The listing builds one solid part. Answer for the finished solid, in the listing's coordinates (mm). Coordinates: 2 decimals unless noted, no trailing zeros. Loops run counter-clockwise (first coordinate to the right, second up) from the corner with the lowest first, then second, coordinate; pieces in that order, holes last. Notation, with made-up numbers: (-37, -4.5) - (16, -4.5) arc R35 ccw to (16, 33.5) - close; hole circle Ø11 at (66, 9.5). An arc over 180 degrees is marked (long way). One line per question, with ' | ' between items.
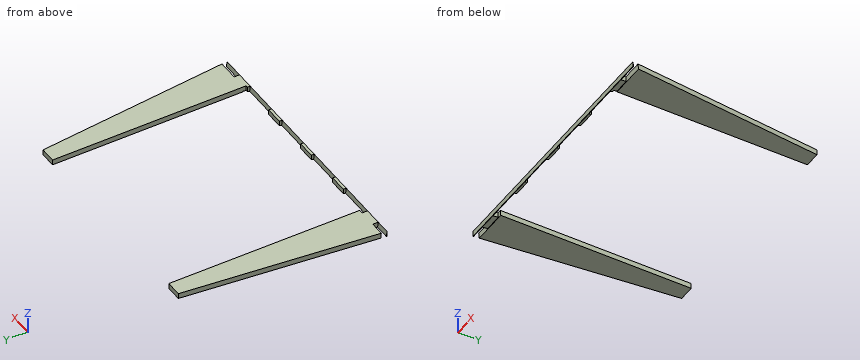
from build123d import *

# Parameters (mm, degrees)
BOSS_EXTRUDE1_DEPTH = 3
CAVITY1_START       = -3.803030659
CAVITY1_OUTLINE_W   = 20
CAVITY1_OUTLINE_H   = 3
CAVITY1_OUTLINE_W_2 = 12.749963879
CAVITY1_OUTLINE_W_3 = 9.250036121
CAVITY1_DEPTH       = 3.331837545
CAVITY1_START_2     = -0.803030659
CAVITY1_2_OUTLINE_W = 10
CAVITY1_2_OUTLINE_H = 3
CAVITY1_2_DEPTH     = 0.331837545


# Read off the part's stored shape, not the designer's step: Cavity1
with BuildPart() as part:
    # Sketch3 → Boss-Extrude1 (new body)
    with BuildSketch(Plane.XY):
        Polygon((-63.438534121, 102.766276007), (-75, -7.839634745), (75, -7.839634745), (63.438534121, 102.766276007), (54.5, 102.766276007), (54.5, -6.233723993), (-54.5, -6.233723993), (-54.5, 102.766276007), align=None)
    extrude(amount=BOSS_EXTRUDE1_DEPTH)

    # Cavity1 outline → Cavity1 (cut)
    with BuildSketch(Plane(origin=(0, 0, 0), x_dir=(1, 0, 0), z_dir=(0, 0.10452846326765304, -0.9945218953682734)).offset(CAVITY1_START)):
        with Locations((43.250036121, 5.983103016)):
            Rectangle(CAVITY1_OUTLINE_W, CAVITY1_OUTLINE_H)
        with Locations((13.250036121, 5.983103016)):
            Rectangle(CAVITY1_OUTLINE_W, CAVITY1_OUTLINE_H)
        with Locations((69.62501806, 5.983103016)):
            Rectangle(CAVITY1_OUTLINE_W_2, CAVITY1_OUTLINE_H)
        with Locations((-16.749963879, 5.983103016)):
            Rectangle(CAVITY1_OUTLINE_W, CAVITY1_OUTLINE_H)
        with Locations((-46.749963879, 5.983103016)):
            Rectangle(CAVITY1_OUTLINE_W, CAVITY1_OUTLINE_H)
        with Locations((-71.37498194, 5.983103016)):
            Rectangle(CAVITY1_OUTLINE_W_3, CAVITY1_OUTLINE_H)
    extrude(amount=CAVITY1_DEPTH, mode=Mode.SUBTRACT)

    # Cavity1 2 outline → Cavity1 2 (cut)
    with BuildSketch(Plane(origin=(0, 0, 0), x_dir=(1, 0, 0), z_dir=(0, 0.10452846326765304, -0.9945218953682734)).offset(CAVITY1_START_2)):
        with Locations((28.250036121, 5.983103016)):
            Rectangle(CAVITY1_2_OUTLINE_W, CAVITY1_2_OUTLINE_H)
        with Locations((58.250036121, 5.983103016)):
            Rectangle(CAVITY1_2_OUTLINE_W, CAVITY1_2_OUTLINE_H)
        with Locations((-1.749963879, 5.983103016)):
            Rectangle(CAVITY1_2_OUTLINE_W, CAVITY1_2_OUTLINE_H)
        with Locations((-31.749963879, 5.983103016)):
            Rectangle(CAVITY1_2_OUTLINE_W, CAVITY1_2_OUTLINE_H)
        with Locations((-61.749963879, 5.983103016)):
            Rectangle(CAVITY1_2_OUTLINE_W, CAVITY1_2_OUTLINE_H)
    extrude(amount=CAVITY1_2_DEPTH, mode=Mode.SUBTRACT)


solid = part.part
Item 1: Find the intervals of material crossed by line 1 (X direction, y = 11.5, z = 1.95); line 2 (Y direction, x = 23.5, z = 0.4); line 3 (X direction, y = 85.5, z = 0.8), in increasing order. Write a range as [from, to].
Taken from the geometry:
line 1: x = [-72.98, -54.5], [54.5, 72.98] | line 2: y = [-7.84, -6.23] | line 3: x = [-65.24, -54.5], [54.5, 65.24]
Item 2: Find section C-C, the plane x = -15. Write down the section's boundary in (y, z), plus the area to 3 significant figures.
Taken from the geometry:
outline: (-7.84, 0) - (-7.52, 0) - (-7.84, 3) - close | area: 0.473 mm2
Item 3: Each of these flat-tipped pins is pushed along its axis until it touches: pin 1 Ø0.9 at (y, z) = (-7, 1.5) entering from +X; pin 2 Ø1.5 at (y, z) = (48.5, 1.5) entering from -X; pin 3 Ø0.9 at (x, z) = (-32.5, 1.5) entering from +Y. Where does it stop, or does it pass through?
Taken from the geometry:
pin 1: stops at x = 63.25 | pin 2: stops at x = -69.19 | pin 3: stops at y = -6.23
Item 4: Find section A-A, the plane y = 39.5. Write down the section's boundary in (x, z), plus the area to 3 significant figures.
Taken from the geometry:
outline: (-70.05, 0) - (-54.5, 0) - (-54.5, 3) - (-70.05, 3) - close; (54.5, 0) - (70.05, 0) - (70.05, 3) - (54.5, 3) - close | area: 93.3 mm2
Item 5: Find section D-D, the plane y = 27.5. Write down the section's boundary in (x, z), plus the area to 3 significant figures.
Taken from the geometry:
outline: (-71.31, 0) - (-54.5, 0) - (-54.5, 3) - (-71.31, 3) - close; (54.5, 0) - (71.31, 0) - (71.31, 3) - (54.5, 3) - close | area: 101 mm2
